```python
from build123d import *

# Parameters (mm, degrees)
EXTRUDE_1_DEPTH     = 8
CHAMFER_1_SIZE      = 0.7
SKETCH_3_W          = 10.8
SKETCH_3_H          = 4.8
SKETCH_3_W_2        = 9.4
SKETCH_3_H_2        = 5.7
CUT_EXTRUDE_1_DEPTH = 7.2
FILLET_1_R          = 0.1
CUT_EXTRUDE_2_REACH = 18.945
SKETCH_4_W          = 5.7
SKETCH_4_H          = 1.2
EXTRUDE_2_REACH     = 18.515
SKETCH_5_W          = 3.9
SKETCH_5_H          = 1.2
EXTRUDE_3_DEPTH     = 1
EXTRUDE_4_REACH     = 18.515
SKETCH_7_W          = 1
SKETCH_7_H          = 1


with BuildPart() as part:
    # ｽｹｯﾁ1 → ﾎﾞｽ - 押し出し1 (new body)
    with BuildSketch(Plane.XY):
        Polygon((0, 6.3), (0, 0), (12.8, 0), (12.8, 6.3), (12.1, 6.3), (12.1, 12.5), (0.7, 12.5), (0.7, 6.3), align=None)
    extrude(amount=EXTRUDE_1_DEPTH)

    # 面取り1
    chamfer_1_edges = [part.edges().sort_by_distance(p)[0] for p in [
        (0.7, 6.3, 4),
        (12.1, 6.3, 4),
    ]]
    chamfer(chamfer_1_edges, length=CHAMFER_1_SIZE - 0.0001)  # a hair under: the kernel refuses the full size

    # ｽｹｯﾁ3 → ｶｯﾄ - 押し出し1 (cut)
    with BuildSketch(Plane.XY.offset(8)):
        with Locations((6.4, 2.4)):
            Rectangle(SKETCH_3_W, SKETCH_3_H)
        with Locations((6.4, 8.65)):
            Rectangle(SKETCH_3_W_2, SKETCH_3_H_2)
    extrude(amount=-CUT_EXTRUDE_1_DEPTH, mode=Mode.SUBTRACT)

    # ﾌｨﾚｯﾄ1
    fillet_1_edges = [part.edges().sort_by_distance(p)[0] for p in [
        (1, 4.8, 4.4),
        (11.8, 4.8, 4.4),
        (11.1, 11.5, 4.4),
        (11.1, 5.8, 4.4),
        (1.7, 5.8, 4.4),
        (1.7, 11.5, 4.4),
    ]]
    fillet(fillet_1_edges, radius=FILLET_1_R)

    # ｶｯﾄ - 押し出し2: up to this face of the body (flat: up to its plane)
    cut_extrude_2_end = Plane(part.part.faces().sort_by_distance((6.4, 11.5, 4.4))[0])
    # ｽｹｯﾁ4 → ｶｯﾄ - 押し出し2 (cut, up to the picked face)
    with BuildSketch(Plane.XZ.offset(-4.8), mode=Mode.PRIVATE) as cut_extrude_2_sk1:
        with Locations((8.95, 1.4)):
            Rectangle(SKETCH_4_W, SKETCH_4_H)
    cut_extrude_2_tool1 = split(extrude(cut_extrude_2_sk1.sketch, amount=-CUT_EXTRUDE_2_REACH, mode=Mode.PRIVATE), bisect_by=cut_extrude_2_end, keep=Keep.BOTH, mode=Mode.PRIVATE)
    add(cut_extrude_2_tool1.solids().sort_by(Axis((8.95, 4.8, 1.4), (0, 1, 0)))[0], mode=Mode.SUBTRACT)

    # ｽｹｯﾁ5 → ﾎﾞｽ - 押し出し2 (add, up to next)
    with BuildSketch(Plane(origin=(0, 5.8, 0), x_dir=(1, 0, 0), z_dir=(0, 1, 0)), mode=Mode.PRIVATE) as extrude_2_sk1:
        with Locations((8.55, -2.6)):
            Rectangle(SKETCH_5_W, SKETCH_5_H)
    extrude_2_tool1 = extrude(extrude_2_sk1.sketch, amount=EXTRUDE_2_REACH, mode=Mode.PRIVATE) - part.part
    add(extrude_2_tool1.solids().sort_by_distance((8.55, 5.8, 2.6))[0])

    # ｽｹｯﾁ6 → ﾎﾞｽ - 押し出し3 (add)
    with BuildSketch(Plane.XY.offset(0.8)):
        with BuildLine():
            Line((4.6, 4.8), (4.6, 0))
            add(Edge.make_bspline(
                [(6.1, 2.3), (6.014846431, 0.686411096), (4.6, 0)],
                knots=[0, 0, 0, 1, 1, 1], degree=2))
            Line((6.1, 2.3), (6.1, 4.8))
            Line((6.1, 4.8), (4.6, 4.8))
        make_face()
    extrude(amount=EXTRUDE_3_DEPTH)

    # ｽｹｯﾁ7 → ﾎﾞｽ - 押し出し4 (add, up to next)
    with BuildSketch(Plane(origin=(0, 5.8, 0), x_dir=(1, 0, 0), z_dir=(0, 1, 0)), mode=Mode.PRIVATE) as extrude_4_sk1:
        with Locations((5.6, -2.5)):
            Rectangle(SKETCH_7_W, SKETCH_7_H)
    extrude_4_tool1 = extrude(extrude_4_sk1.sketch, amount=EXTRUDE_4_REACH, mode=Mode.PRIVATE) - part.part
    add(extrude_4_tool1.solids().sort_by_distance((5.6, 5.8, 2.5))[0])


solid = part.part
```
Source: CAD feature listing. Evaluate the final solid. Frame: model axes, mm. A direction names the side the tool comes from. Give positions to 0.01 mm unless a question says otherwise; leave off trailing zeros. Order: outer loops, then holes, each group sorted by start corner. A loop starts at its lowest first (then second) coordinate and runs counter-clockwise, first axis right, second up.
(1) Section query C-C (x = 2). Return the cut outline in (y, z).
(2) Access query for faces 1 (the face through (8, 7, 0.8)), 2 (the face through (0.7, 10, 4)), 3 (the face through (4.6, 2, 1)), 4 (the face through (5.1, 8.6, 2.5)). Directions: +Z, -Z, +X, -X, +Y, -Y. A direction counts if a zero-diameter tool reaches every point of the face in a straight line with its end or side. Return the directions, or none.
(3) Section query A-A (y = 10.5). Return the cut outline in (x, z), plus the area to 3 significant figures.
(4) Material intervals for line 1 along Y through (x, z) = (7.5, 7.25); line 2 along Z through (x, y) = (11.25, 10.25); line 3 along X through (y, z) = (4.25, 3.25), sorted ascending.
(5) Contact query for flat-ended pins moving along their axis: P1, Ø2, axis at x = 7, z = 3, coming from the -Y side; P2, Ø0.5, axis at y = 10, z = 2.5, coming from the -X side; P3, Ø1.3, axis at y = 9, z = 2.5, coming from the +X side. Output: stop coordinate, or through.
(6) Section query D-D (y = 5.5). Return the cut outline in (x, z), plus the area to 3 significant figures.
(7) Pull-direction query (Z, two-part tool) for faces 5 (the face through (5.6, 8.6, 3)), 6 (the face through (5.6, 8.6, 2)), 7 (the face through (6, 4.8, 4)); classes: +Z half, -Z half, draft (parallel to the pull), parting line (faces both ways), or undercut.
Outcome:
1. outline: (0, 0) - (12.5, 0) - (12.5, 8) - (11.5, 8) - (11.5, 0.8) - (5.8, 0.8) - (5.8, 8) - (4.8, 8) - (4.8, 0.8) - (0, 0.8) - close
2. face 1: none
2. face 2: +Z, -Z, -X, +Y
2. face 3: +Z, -Y
2. face 4: +Z
3. outline: (0.7, 0) - (12.1, 0) - (12.1, 8) - (11.1, 8) - (11.1, 2) - (11.8, 2) - (11.8, 0.8) - (1.7, 0.8) - (1.7, 8) - (0.7, 8) - close; (5.1, 2) - (6.1, 2) - (6.1, 3) - (5.1, 3) - close; (6.6, 2) - (10.5, 2) - (10.5, 3.2) - (6.6, 3.2) - close
3. area: 28.4 mm2
4. line 1: y = 4.8 to 5.8, 11.5 to 12.5
4. line 2: z = 0 to 0.8, 2 to 8
4. line 3: x = 0 to 1, 11.8 to 12.8
5. P1: stops at y = 4.8
5. P2: stops at x = 0.7
5. P3: stops at x = 12.1
6. outline: (0, 0) - (12.8, 0) - (12.8, 8) - (0, 8) - close; hole (6.1, 0.8) - (11.8, 0.8) - (11.8, 2) - (6.1, 2) - close
6. area: 95.6 mm2
7. face 5: +Z half
7. face 6: undercut
7. face 7: draft
